Source: CAD feature listing. Evaluate the final solid. Frame: model axes, mm. Give positions to 0.01 mm unless a question says otherwise; leave off trailing zeros. Loops run counter-clockwise (first coordinate to the right, second up) from the corner with the lowest first, then second, coordinate; pieces in that order, holes last. Notation, with made-up numbers: M 1.5,76 L 23.5,76 A15 cw 23.5,100 Z; hole C -2.75,-31.5 d8. An arc over 180 degrees is marked long. Answer in a Markdown table with one row per item.
```python
from build123d import *

# Parameters (mm, degrees)
SKETCH1_R           = 12.7
BOSS_EXTRUDE1_DEPTH = 279.4
SKETCH2_R           = 8.89
CUT_EXTRUDE1_DEPTH  = 280.9766776
SKETCH3_R           = 10.033
CUT_EXTRUDE2_DEPTH  = 12.7
CUT_EXTRUDE3_START  = -12.192
SKETCH4_R           = 12.7
SKETCH4_R_2         = 10.16
CUT_EXTRUDE3_DEPTH  = 12.192
FILLET1_R           = 1.27
CHAMFER1_SIZE       = 1.27
FILLET2_R           = 0.635
CHAMFER2_SIZE       = 1.27


with BuildPart() as part:
    # Sketch1 → Boss-Extrude1 (new body)
    with BuildSketch(Plane.XY):
        Circle(SKETCH1_R)
    extrude(amount=BOSS_EXTRUDE1_DEPTH)

    # Sketch2 → Cut-Extrude1 (cut, through all)
    with BuildSketch(Plane(origin=(0, 0, 0), x_dir=(-1, 0, 0), z_dir=(0, 0, -1))):
        Circle(SKETCH2_R)
    extrude(amount=-CUT_EXTRUDE1_DEPTH, mode=Mode.SUBTRACT)

    # Sketch3 → Cut-Extrude2 (cut)
    with BuildSketch(Plane(origin=(0, 0, 0), x_dir=(-1, 0, 0), z_dir=(0, 0, -1))):
        Circle(SKETCH3_R)
    extrude(amount=-CUT_EXTRUDE2_DEPTH, mode=Mode.SUBTRACT)

    # Sketch4 → Cut-Extrude3 (cut)
    with BuildSketch(Plane.XY.offset(279.4).offset(CUT_EXTRUDE3_START)):
        Circle(SKETCH4_R)
        Circle(SKETCH4_R_2, mode=Mode.SUBTRACT)
    extrude(amount=CUT_EXTRUDE3_DEPTH, mode=Mode.SUBTRACT)

    # Fillet1
    fillet1_edges = [part.edges().sort_by_distance(p)[0] for p in [
        (-10.16, 0, 267.208),
    ]]
    fillet(fillet1_edges, radius=FILLET1_R)

    # Chamfer1
    chamfer1_edges = [part.edges().sort_by_distance(p)[0] for p in [
        (10.033, 0, 0),
    ]]
    chamfer(chamfer1_edges, length=CHAMFER1_SIZE)

    # Fillet2
    fillet2_edges = [part.edges().sort_by_distance(p)[0] for p in [
        (10.033, 0, 12.7),
    ]]
    fillet(fillet2_edges, radius=FILLET2_R)

    # Chamfer2
    chamfer2_edges = [part.edges().sort_by_distance(p)[0] for p in [
        (-10.16, 0, 279.4),
    ]]
    chamfer(chamfer2_edges, length=CHAMFER2_SIZE - 0.0001)  # a hair under: the kernel refuses the full size


solid = part.part
```
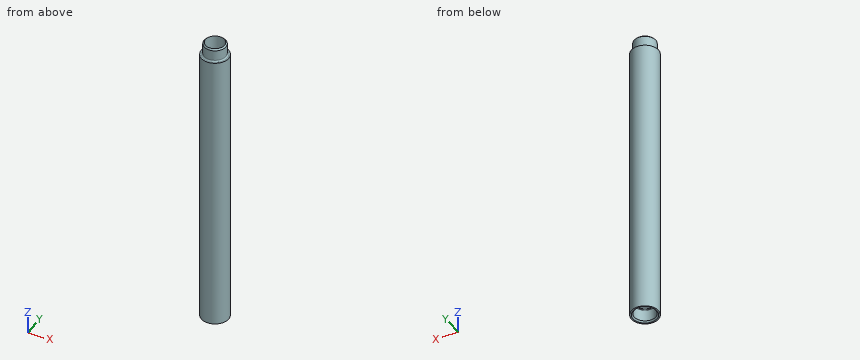
1) Section C-C, the plane z = 26. Return loops of the section in (x, y).
Reply:
| item | result |
|---|---|
| outline | C 0,0 d25.4; hole C 0,0 d17.78 |
2) Pin query (flat end, axial travel): pin 1 Ø5 at (x, z) = (3.5, 141) entering from -Y; pin 2 Ø12 at (x, y) = (0, 0) entering from +Z; pin 3 Ø10 at (x, z) = (8, 150.5) entering from -Y; pin 4 Ø4 at (x, y) = (-3.5, -6.5) entering from -Z. Return the tip coordinate at first contact, or that it passes through.
Reply:
| item | result |
|---|---|
| pin 1 | stops at y = -12.66 |
| pin 2 | passes through |
| pin 3 | stops at y = -12.34 |
| pin 4 | stops at z = 12.7 |
3) Material intervals for L1, parallel to Y at x = 0, z = 8; L2, parallel to X at y = -0.75, z = 247; L3, parallel to X at y = -6, z = 187, sorted ascending.
Reply:
| item | result |
|---|---|
| L1 | y = -12.7 to -10.03, 10.03 to 12.7 |
| L2 | x = -12.68 to -8.86, 8.86 to 12.68 |
| L3 | x = -11.19 to -6.56, 6.56 to 11.19 |
